Verification items for the finished model (mm, model axes). Face numbers are marked on the shaded views. Coordinates: 2 decimals unless noted, no trailing zeros. Order: outer loops, then holes, each group sorted by start corner. A loop starts at its lowest first (then second) coordinate and runs counter-clockwise, first axis right, second up. Notation, with made-up numbers: (78.5, -36.75) -> (109.5, -36.75) arc R27 ccw to (109.5, -20.75) -> close; hole circle Ø4 at (77.5, 28). An arc over 180 degrees is marked (long way). Answer as CSV lines item,"result".
```python
from build123d import *

# Parameters (mm, degrees)
F0_R     = 1.5
F1_DEPTH = 6
F2_W     = 50.6
F2_H     = 86.6
F2_R     = 1.5
F3_DEPTH = 6
F4_R     = 1.5
F5_DEPTH = 2


with BuildPart() as f1:
    # F0 (on Top) → F1 (new body)
    with BuildSketch(Plane.XY):
        with BuildLine():
            Line((-25, -48), (25, -48))
            ThreePointArc((25, -48), (28.535534, -46.535534), (30, -43))
            Line((30, -43), (30, 43))
            ThreePointArc((30, 43), (28.535534, 46.535534), (25, 48))
            Line((25, 48), (-27, 48))
            Line((-27, 48), (-30, 48))
            Line((-30, 48), (-30, 43))
            Line((-30, 43), (-30, -43))
            ThreePointArc((-30, -43), (-28.535534, -46.535534), (-25, -48))
        make_face()
        with Locations((-22, -36.08)):
            Circle(F0_R, mode=Mode.SUBTRACT)
        with Locations((22, -36.08)):
            Circle(F0_R, mode=Mode.SUBTRACT)
        with Locations((-22, 40)):
            Circle(F0_R, mode=Mode.SUBTRACT)
        with Locations((22, 40)):
            Circle(F0_R, mode=Mode.SUBTRACT)
    extrude(amount=F1_DEPTH)

    # F2 (on face) → F3 (cut)
    with BuildSketch(Plane.XY.offset(6)):
        Rectangle(F2_W, F2_H)
        with Locations((-22, -36.08)):
            Circle(F2_R, mode=Mode.SUBTRACT)
        with Locations((22, -36.08)):
            Circle(F2_R, mode=Mode.SUBTRACT)
        with Locations((-22, 40)):
            Circle(F2_R, mode=Mode.SUBTRACT)
        with Locations((22, 40)):
            Circle(F2_R, mode=Mode.SUBTRACT)
    extrude(amount=-F3_DEPTH, mode=Mode.SUBTRACT)

    # F4 (on face) → F5 (join)
    with BuildSketch(Plane(origin=(0, 0, 0), x_dir=(1, 0, 0), z_dir=(0, 0, -1))):
        with BuildLine():
            Line((-30, 43), (-30, -48))
            Line((-30, -48), (25, -48))
            ThreePointArc((25, -48), (28.535534, -46.535534), (30, -43))
            Line((30, -43), (30, 43))
            ThreePointArc((30, 43), (28.535534, 46.535534), (25, 48))
            Line((25, 48), (-25, 48))
            ThreePointArc((-25, 48), (-28.535534, 46.535534), (-30, 43))
        make_face()
        with Locations((-22, -40)):
            Circle(F4_R, mode=Mode.SUBTRACT)
        with Locations((22, -40)):
            Circle(F4_R, mode=Mode.SUBTRACT)
        with Locations((-22, 36.08)):
            Circle(F4_R, mode=Mode.SUBTRACT)
        with Locations((22, 36.08)):
            Circle(F4_R, mode=Mode.SUBTRACT)
    extrude(amount=F5_DEPTH)


solid = f1.part
```
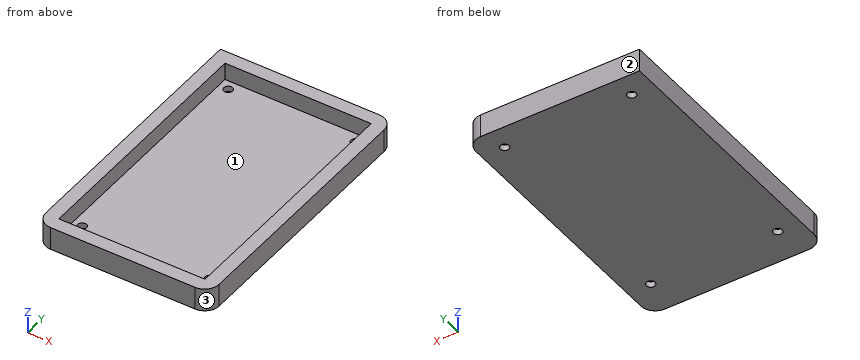
Item 1: Release check for a two-part mould opening along X. For the marked faces 1, 2 and 3 record: +X half, -X half, draft (parallel to the pull), parting line (faces both ways), or undercut.
Answer list:
face 1,"undercut"
face 2,"draft"
face 3,"+X half"
Item 2: Section check B-B, the plane x = 22. Record the boundary of the cut face in (y, z).
Answer list:
outline,"(-48, -2) -> (-37.58, -2) -> (-37.58, 0) -> (-43.3, 0) -> (-43.3, 6) -> (-48, 6) -> close; (-34.58, -2) -> (38.5, -2) -> (38.5, 0) -> (-34.58, 0) -> close; (41.5, -2) -> (48, -2) -> (48, 6) -> (43.3, 6) -> (43.3, 0) -> (41.5, 0) -> close"
Item 3: Section check C-C, the plane y = 34.5. Record the boundary of the cut face in (x, z).
Answer list:
outline,"(-30, -2) -> (30, -2) -> (30, 6) -> (25.3, 6) -> (25.3, 0) -> (-25.3, 0) -> (-25.3, 6) -> (-30, 6) -> close"
Item 4: Thickness scan on line 1 (Y direction, x = -22, z = -0.55); line 2 (X direction, y = -26.5, z = 3); line 3 (Y direction, x = -8, z = 1.5). Record the ranges inside material, lowest first.
Answer list:
line 1,"-48 to -37.58, -34.58 to 38.5, 41.5 to 48"
line 2,"-30 to -25.3, 25.3 to 30"
line 3,"-48 to -43.3, 43.3 to 48"
Item 5: Section check A-A, the plane y = -36.08. Record the boundary of the cut face in (x, z).
Answer list:
outline,"(-30, -2) -> (-23.5, -2) -> (-23.5, 0) -> (-25.3, 0) -> (-25.3, 6) -> (-30, 6) -> close; (-20.5, -2) -> (20.5, -2) -> (20.5, 0) -> (-20.5, 0) -> close; (23.5, -2) -> (30, -2) -> (30, 6) -> (25.3, 6) -> (25.3, 0) -> (23.5, 0) -> close"
Item 6: Section check D-D, the plane z = 4. Record the boundary of the cut face in (x, y).
Answer list:
outline,"(-30, -43) arc R5 ccw to (-25, -48) -> (25, -48) arc R5 ccw to (30, -43) -> (30, 43) arc R5 ccw to (25, 48) -> (-30, 48) -> close; hole (-25.3, -43.3) -> (25.3, -43.3) -> (25.3, 43.3) -> (-25.3, 43.3) -> close"
